```python
from build123d import *

# Parameters (mm, degrees)
SKETCH_1_R      = 2
EXTRUDE_1_DEPTH = 0.5
EXTRUDE_2_DEPTH = 3
SKETCH_4_W      = 7
SKETCH_4_H      = 0.5
EXTRUDE_3_DEPTH = 8
F_2_5MM_1_D     = 2.5
FILLET_1_R      = 2


with BuildPart() as part:
    # 草圖1 → 填料-伸長1 (new body)
    with BuildSketch(Plane.XY):
        with BuildLine():
            Line((-4, 0), (4, 0))
            Line((4, 0), (2.947629603, 5.558103683))
            ThreePointArc((2.947629603, 5.558103683), (0, 8), (-2.947629603, 5.558103683))
            Line((-2.947629603, 5.558103683), (-4, 0))
        make_face()
        with Locations((0, 5)):
            Circle(SKETCH_1_R, mode=Mode.SUBTRACT)
    extrude(amount=EXTRUDE_1_DEPTH)

    # 草圖1<3> → 填料-伸長2 (add)
    with BuildSketch(Plane.XY):
        Polygon((-3.905330086, 0.5), (-4, 0), (4, 0), (3.905330086, 0.5), align=None)
    extrude(amount=-EXTRUDE_2_DEPTH)

    # 鏡射1: part across plane


with BuildPart() as part_1:
    add(part.part)
    add(part.part.mirror(Plane.XY.offset(-3)))

    # 草圖4 → 填料-伸長3 (add, symmetric)
    with BuildSketch(Plane(origin=(0, 0, 0), x_dir=(0, 0, -1), z_dir=(1, 0, 0))):
        with Locations((3, 0.25)):
            Rectangle(SKETCH_4_W, SKETCH_4_H)
    extrude(amount=EXTRUDE_3_DEPTH, both=True)

    # Ø2.5mm 定位孔1 (through all)
    with Locations(Plane(origin=(0, 0.5, 0), x_dir=(1, 0, 0), z_dir=(0, 1, 0))):
        with Locations((-6, 3), (6, 3)):
            Hole(F_2_5MM_1_D / 2)

    # 圓角1
    fillet_1_edges = [part_1.edges().sort_by_distance(p)[0] for p in [
        (-8, 0.25, 0.5),
        (-8, 0.25, -6.5),
        (8, 0.25, 0.5),
        (8, 0.25, -6.5),
    ]]
    fillet(fillet_1_edges, radius=FILLET_1_R)


solid = part_1.part
```
Check sheet for the modelled part. Datum: model origin and axes. Units: mm. A direction names the side the tool comes from. Give positions to 0.01 mm unless a question says otherwise; leave off trailing zeros. Write each loop counter-clockwise with the first axis right and the second up, starting at its lowest first coordinate (ties: lowest second). Pieces come first, ordered by that corner, then holes. Notation, with made-up numbers: (19.25, 10.25) - (24.25, 10.25) arc R30 ccw to (24.25, 45.25) - close; hole circle Ø10 at (1.25, 1). An arc over 180 degrees is marked (long way). Answer as a JSON object with one key per item and string values. Group by question number.
1) Release check for a two-part mould opening along X. For faces 3 (the face through (-0.26, 6.983, 0.246)), 4 (the face through (0.1, 8, -6.2)), 5 (the face through (0, 2, 0.5)) record: pulls with the +X half, pulls with the -X half, needs draft (parallel to the pull), parting line crosses it, or undercut.
2) Thickness scan on probe 1 along Z at (x, y) = (1.25, 2); probe 2 along Y at (x, z) = (0, 0.3); probe 3 along Y at (x, z) = (-6.25, -4.5). Record the ranges inside material, lowest first. Write a range as from..to.
3) Sectioned sample at B-B (x = 5.25). Record the cut outline in (y, z).
4) Depth check by flat-ended pin: P1, Ø2, axis at x = 3.5, z = -3, coming from the +Y side. Enter the tip coordinate at first touch or a pass-through.
5) Access from +Z, -Z, +X, -X, +Y, -Y to the whole of each face (thin tool, end or side, straight path). Record for faces 1 (the face through (-0.26, 6.983, -6.246)), 2 (the face through (-0.1, 2.6, -6)).
6) Sectioned sample at D-D (x = -1.5). Record the cut outline in (y, z), then the cut area to 3 significant figures.
7) Sectioned sample at C-C (y = 6.25). Record the cut outline in (x, z), then the cut area to 3 significant figures.
8) Sectioned sample at A-A (z = -3). Record the cut outline in (x, y).
Geometry results:
{
 "1": {"face 3": "undercut", "face 4": "parting line crosses it", "face 5": "needs draft"},
 "2": {"probe 1": "z = -6.5..-6, 0..0.5", "probe 2": "y = 0..3, 7..8", "probe 3": "y = 0..0.5"},
 "3": {"outline": "(0, -6.5) - (0.5, -6.5) - (0.5, -4) - (0, -4) - close; (0, -2) - (0.5, -2) - (0.5, 0.5) - (0, 0.5) - close"},
 "4": {"P1": "stops at y = 0.5"},
 "5": {"face 1": "+Z, -Z", "face 2": "+X, -X, +Y"},
 "6": {"outline": "(0, -6.5) - (3.68, -6.5) - (3.68, -6) - (0.5, -6) - (0.5, 0) - (3.68, 0) - (3.68, 0.5) - (0, 0.5) - close; (6.32, -6.5) - (7.6, -6.5) - (7.6, -6) - (6.32, -6) - close; (6.32, 0) - (7.6, 0) - (7.6, 0.5) - (6.32, 0.5) - close", "area": "7.95 mm^2"},
 "7": {"outline": "(-2.73, -6.5) - (-1.56, -6.5) - (-1.56, -6) - (-2.73, -6) - close; (-2.73, 0) - (-1.56, 0) - (-1.56, 0.5) - (-2.73, 0.5) - close; (1.56, -6.5) - (2.73, -6.5) - (2.73, -6) - (1.56, -6) - close; (1.56, 0) - (2.73, 0) - (2.73, 0.5) - (1.56, 0.5) - close", "area": "2.33 mm^2"},
 "8": {"outline": "(-8, 0) - (-7.25, 0) - (-7.25, 0.5) - (-8, 0.5) - close; (-4.75, 0) - (4.75, 0) - (4.75, 0.5) - (-4.75, 0.5) - close; (7.25, 0) - (8, 0) - (8, 0.5) - (7.25, 0.5) - close"}
}
